from build123d import *

# Parameters (mm, degrees)
F1_DEPTH    = 584.2
F2_T1_DEPTH = 584.2
F2_T3_DEPTH = 600.075
F3_R        = 3.175
F4_DEPTH    = 1.5875
F5_R        = 3.175
F6_DEPTH    = 1.5875
F7_R        = 3.175
F8_DEPTH    = 1.5875
F9_R        = 3.175
F10_DEPTH   = 1.5875
F11_R       = 8.0645
F12_DEPTH   = 1.5875


# Not quite as in the source:
# - a fillet or chamfer that OpenCascade refuses, or shapes differently, is made with other operations: its cross-section is extruded or revolved along the edge and cut away or added


with BuildPart() as f1:
    # F0 (on Top) → F1 (new body)
    with BuildSketch(Plane.XY):
        Polygon((-5.119352553, 3.4975720825), (-5.119352553, 33.6600720825), (-6.706852553, 33.6600720825), (-6.706852553, 1.9100720825), (25.043147447, 1.9100720825), (25.043147447, 3.4975720825), align=None)
    extrude(amount=F1_DEPTH)

    # F2: fillet of radius 3.175 on 2 edges, made by hand

    # F2_s2 → F2_t1 (join)
    with BuildSketch(Plane.XY):
        with BuildLine():
            add(Edge.make_bspline(
                [(-1.944352553, 3.4975720825), (-5.119352553, 3.4975720825), (-5.119352553, 6.6725720825)],
                knots=[0, 0, 0, 1, 1, 1], degree=2, weights=[1, 1, 1]))
            Line((-5.119352553, 6.6725720825), (-5.119352553, 3.4975720825))
            Line((-5.119352553, 3.4975720825), (-1.944352553, 3.4975720825))
        make_face()
    extrude(amount=F2_T1_DEPTH)

    # F2_s4 → F2_t3 (cut)
    with BuildSketch(Plane.XY.offset(-7.9375)):
        with BuildLine():
            add(Edge.make_bspline(
                [(-6.706852553, 5.0850720825), (-6.706852553, 1.9100720825), (-3.531852553, 1.9100720825)],
                knots=[0, 0, 0, 1, 1, 1], degree=2, weights=[1, 1, 1]))
            Line((-3.531852553, 1.9100720825), (-6.706852553, 1.9100720825))
            Line((-6.706852553, 1.9100720825), (-6.706852553, 5.0850720825))
        make_face()
    extrude(amount=F2_T3_DEPTH, mode=Mode.SUBTRACT)

    # F3 (on face) → F4 (cut)
    with BuildSketch(Plane.YZ.offset(-5.119352553)):
        with Locations((20.1663220825, 12.7)):
            Circle(F3_R)
        with Locations((20.1663220825, 571.5)):
            Circle(F3_R)
    extrude(amount=-F4_DEPTH, mode=Mode.SUBTRACT)

    # F5 (on face) → F6 (cut)
    with BuildSketch(Plane(origin=(0, 3.4975720825, 0), x_dir=(-1, 0, 0), z_dir=(0, 1, 0))):
        with Locations((-11.549397447, 12.7)):
            Circle(F5_R)
        with Locations((-11.549397447, 571.5)):
            Circle(F5_R)
    extrude(amount=-F6_DEPTH, mode=Mode.SUBTRACT)

    # F7 (on face) → F8 (cut)
    with BuildSketch(Plane.XZ.offset(-1.9100720825)):
        with Locations((5.993147447, 508)):
            Circle(F7_R)
        with Locations((18.693147447, 508)):
            Circle(F7_R)
    extrude(amount=-F8_DEPTH, mode=Mode.SUBTRACT)

    # F9 (on face) → F10 (cut)
    with BuildSketch(Plane.XZ.offset(-1.9100720825)):
        with Locations((10.755647447, 38.1)):
            Circle(F9_R)
        with Locations((10.755647447, 50.8)):
            Circle(F9_R)
    extrude(amount=-F10_DEPTH, mode=Mode.SUBTRACT)

    # F11 (on face) → F12 (cut)
    with BuildSketch(Plane.XZ.offset(-1.9100720825)):
        with Locations((5.993147447, 76.2)):
            Circle(F11_R)
    extrude(amount=-F12_DEPTH, mode=Mode.SUBTRACT)


solid = f1.part
Build history of the part. All positions in model axes, mm. A direction names the side the tool comes from. Round coordinates to 2 decimals unless told otherwise and drop trailing zeros. Use CSV: the item, a comma, the result in double quotes. Start each with the question number.
Q1. Which spindle directions (+Z, -Z, +X, -X, +Y, -Y) get a long thin tool onto all of the face, cutting with end or side? Do faces 4 (the face through (12, 3.498, 288)), 5 (the face through (-6.707, 20, 288)). Say none if no direction does.
Q2. Mould opens along X. For faces 1 (the face through (9.714, 2.693, 69.045)), 2 (the face through (1, 3, 584.2)), 3 (the face through (-5.119, 20, 288)) say: +X half, -X half, draft (parallel to the pull), parting line (faces both ways), or undercut.
Q3. Drill centre lines: L1, parallel to X at y = 8.5, z = 475; L2, parallel to Y at x = 3, z = 390; L3, parallel to Y at x = -3, z = 300.5. Where is each one in solid material? Low to high.
Q4. Flat gauge pins, fed straight in: pin 1 Ø12 at (x, z) = (17, 468) entering from +Y; pin 2 Ø12 at (y, z) = (15.5, 198.5) entering from +X; pin 3 Ø4 at (y, z) = (20.17, 571.5) entering from -X. Where does each tip first touch, or does it go through?
Solutions:
1,face 4,"+Z, -Z, +X, +Y"
1,face 5,"+Z, -Z, -X, +Y, -Y"
2,face 1,"undercut"
2,face 2,"draft"
2,face 3,"+X half"
3,L1,"x = -6.71 to -5.12"
3,L2,"y = 1.91 to 3.5"
3,L3,"y = 1.91 to 3.6"
4,pin 1,"stops at y = 3.5"
4,pin 2,"stops at x = -5.12"
4,pin 3,"passes through"
